Geometry: final body of the model. Coordinates: model frame, mm. A direction names the side the tool comes from. Round coordinates to 2 decimals unless told otherwise and drop trailing zeros. Loops run counter-clockwise (first coordinate to the right, second up) from the corner with the lowest first, then second, coordinate; pieces in that order, holes last. Notation, with made-up numbers: M 79,-10.5 L 107,-10.5 A11 ccw 107,2.5 Z; hole C 75.5,58.25 d4. An arc over 180 degrees is marked long. Answer as a JSON object with one key per item and string values.
from build123d import *

# Parameters (mm, degrees)
PAD027_DEPTH    = 1.8
SKETCH062_R     = 3.3
PAD028_DEPTH    = 8.2
FILLET_R        = 0.5
SKETCH101_R     = 0.05
POCKET045_DEPTH = 4
POCKET045_TAPER = -60


with BuildPart() as part:
    # Sketch061 → Pad027 (new body)
    with BuildSketch(Plane.XY):
        with BuildLine():
            Line((-12.88, -25.84), (-12.88, -31.74))
            ThreePointArc((-12.88, -31.74), (-11.752361, -34.462361), (-9.03, -35.59))
            Line((-9.03, -35.59), (-4.78, -35.59))
            ThreePointArc((-4.78, -35.59), (-3.71934, -35.15066), (-3.28, -34.09))
            Line((-3.28, -34.09), (-3.28, -23.49))
            ThreePointArc((-3.28, -23.49), (-3.71934, -22.42934), (-4.78, -21.99))
            Line((-4.78, -21.99), (-9.03, -21.99))
            ThreePointArc((-9.03, -21.99), (-11.752361, -23.117639), (-12.88, -25.84))
        make_face()
    extrude(amount=-PAD027_DEPTH)

    # Sketch062 → Pad028 (join)
    with BuildSketch(Plane.XY.offset(-1.8)):
        with Locations((-7.58, -28.79)):
            Circle(SKETCH062_R)
    extrude(amount=-PAD028_DEPTH)

    # Fillet
    fillet_edges = [part.edges().sort_by_distance(p)[0] for p in [
        (-12.88, -28.79, 0),
        (-11.752361, -34.462361, 0),
        (-6.905, -35.59, 0),
        (-3.71934, -35.15066, 0),
        (-3.28, -28.79, 0),
        (-3.71934, -22.42934, 0),
        (-6.905, -21.99, 0),
        (-11.752361, -23.117639, 0),
    ]]
    fillet(fillet_edges, radius=FILLET_R)

    # Sketch101 → Pocket045 (cut)
    with BuildSketch(Plane.XY.offset(-2)):
        with Locations((-8.08, -28.79)):
            Circle(SKETCH101_R)
    extrude(amount=POCKET045_DEPTH, taper=POCKET045_TAPER, mode=Mode.SUBTRACT)


with BuildPart() as part_1:
    # Body008 placement: moved
    add(part.part.moved(Location((0, 0, 26.4))))


solid = part_1.part
1) Pull-direction query (Y, two-part tool) for faces 1 (the flat face through (-8, -29, 16.4)), 2 (the conical face through (-8.277, -28.61, 24.525)), 3 (the cylindrical face through (-11.782, -34.432, 25.259)), 4 (the flat face through (-7, -21.99, 25)); classes: +Y half, -Y half, draft (parallel to the pull), parting line (faces both ways), or undercut.
Results:
{"face 1": "draft", "face 2": "undercut", "face 3": "-Y half", "face 4": "+Y half"}
2) Section query A-A (z = 23.5). Return the cut outline in (x, y), and give its area (3 significant figures).
Results:
{"outline": "C -7.58,-28.79 d6.6", "area": "34.2 mm2"}
3) Ray query, line 1 (Z direction, x = -10.5, y = -26); line 2 (Y direction, x = -9.5, z = 25.75); line 3 (Y direction, x = -7.5, z = 23.5). Return the intervals inside material, ascending.
Results:
{"line 1": "24.6 to 26.4", "line 2": "-35.56 to -30.71, -26.87 to -22.02", "line 3": "-32.09 to -25.49"}
4) Pin query (flat end, axial travel): P1, Ø2, axis at x = -6, z = 18, coming from the -Y side; P2, Ø1.5, axis at y = -28.5, z = 22, coming from the +X side; P3, Ø3, axis at y = -25, z = 20.5, coming from the -X side. Return the tip coordinate at first contact, or that it passes through.
Results:
{"P1": "y = -32.04", "P2": "x = -4.28", "P3": "x = -9.96"}
5) Reachability of faces 5 (the flat face through (-9, -32, 24.6)), 6 (the cylindrical face through (-3.73, -35.16, 25.26)) from +Z, -Z, +X, -X, +Y, -Y: full face, straight path, thin tool, end or side. Return the list, or none.
Results:
{"face 5": "-Z", "face 6": "+Z, -Z, +X, -Y"}
